The listing builds one solid part. Answer for the finished solid, in the listing's coordinates (mm). A direction names the side the tool comes from. Round coordinates to 2 decimals unless told otherwise and drop trailing zeros. Write each loop counter-clockwise with the first axis right and the second up, starting at its lowest first coordinate (ties: lowest second). Pieces come first, ordered by that corner, then holes. Notation, with made-up numbers: (48.25, -24) - (58.25, -24) arc R35 ccw to (58.25, 10) - close; hole circle Ø9 at (4.5, 36.5). An arc over 180 degrees is marked (long way). Answer in a Markdown table with one row per item.
from build123d import *

# Parameters (mm, degrees)
F1_DEPTH = 30
F2_R     = 29.99999
F3_R     = 10


# Not quite as in the source:
# - a fillet or chamfer is up to 0.001 mm smaller than in the source, because OpenCascade refuses the exact size


with BuildPart() as f1:
    # F0 (on Front) → F1 (new body, symmetric)
    with BuildSketch(Plane.XZ):
        with BuildLine():
            Line((30, -5), (30, 75))
            Line((30, 75), (-30, 75))
            Line((-30, 75), (-30, -5))
            Line((-30, -5), (-60, -5))
            Line((-60, -5), (-60, -45))
            ThreePointArc((-60, -45), (0, -59.0661337755), (60, -45))
            Line((60, -45), (60, -5))
            Line((60, -5), (30, -5))
        make_face()
    extrude(amount=F1_DEPTH, both=True)

    # F2 (radius 30 in the source; OpenCascade refuses exactly that, so slightly less here)
    f2_edges = [f1.edges().sort_by_distance(p)[0] for p in [
        (30, 0, 75),
        (-30, 0, 75),
    ]]
    fillet(f2_edges, radius=F2_R)

    # F3
    f3_edges = [f1.edges().sort_by_distance(p)[0] for p in [
        (30, -30, 20.000005),
        (21.213206, -30, 66.213206),
        (45, -30, -5),
        (0, -30, 75),
        (60, -30, -25),
        (-21.213206, -30, 66.213206),
        (0, -30, -59.066134),
        (-30, -30, 20.000005),
        (-60, -30, -25),
        (-45, -30, -5),
        (30, 30, 20.000005),
        (30, 0, 45.00001),
        (30, 0, -5),
        (60, 30, -25),
        (60, 0, -5),
        (60, 0, -45),
        (-30, 0, -5),
        (-45, 30, -5),
        (-60, 0, -5),
        (21.213206, 30, 66.213206),
        (45, 30, -5),
        (0, 30, 75),
        (-21.213206, 30, 66.213206),
        (0, 30, -59.066134),
        (-30, 30, 20.000005),
        (-60, 30, -25),
        (-60, 0, -45),
    ]]
    fillet(f3_edges, radius=F3_R)


solid = f1.part
(1) Find the intervals of material crossed by line 1 (X direction, y = -9.5, z = 39.5); line 2 (Z direction, x = 48.5, y = 13.5); line 3 (X direction, y = 6, z = -43), in increasing order.
Checked values:
| item | result |
|---|---|
| line 1 | x = -30 to 30 |
| line 2 | z = -50.05 to -5 |
| line 3 | x = -58.99 to 58.99 |
(2) Section B-B (z = 13) is taken. Give the vertices of the cut face in (x, y), and give its area (3 significant figures).
Checked values:
| item | result |
|---|---|
| outline | (-30, -20) arc R10 ccw to (-20, -30) - (20, -30) arc R10 ccw to (30, -20) - (30, 20) arc R10 ccw to (20, 30) - (-20, 30) arc R10 ccw to (-30, 20) - close |
| area | 3,510 mm2 |
(3) Flat-ended cylindrical pins translate along their axes: pin 1 (5 mm diameter, centred on x = 24.5, y = 5.5, fed in from +Z); pin 2 (1 mm diameter, centred on x = 2, y = -11.5, fed in from +Z); pin 3 (3 mm diameter, centred on x = -43, y = -6, fed in from +Z). Find the tip coordinate at first contact, or state that the pin passes through.
Checked values:
| item | result |
|---|---|
| pin 1 | stops at z = 65.4 |
| pin 2 | stops at z = 74.96 |
| pin 3 | stops at z = -5 |
(4) For faces 1 (the cylindrical face through (-27.15, 26.99, 24.72)), 2 (the flat face through (30, 0, 25)), 3 (the cylindrical face through (27.15, -26.99, 25.28)), 4 (the cylindrical face through (44.93, 27.15, -8.01)), determine the directions among +Z, -Z, +X, -X, +Y, -Y from which every point of the face is accessible in a straight line to the end or side of a thin tool.
Checked values:
| item | result |
|---|---|
| face 1 | +Z, -X, +Y |
| face 2 | +Z, +X, +Y, -Y |
| face 3 | +Z, +X, -Y |
| face 4 | +Z, +X, +Y |
